Model file for the job. Use its own axes, mm. Give positions to 0.01 mm unless a question says otherwise; leave off trailing zeros. Order: outer loops, then holes, each group sorted by start corner. A loop starts at its lowest first (then second) coordinate and runs counter-clockwise, first axis right, second up. Notation, with made-up numbers: (8, 79.25) - (41, 79.25) arc R10 ccw to (41, 92.25) - close; hole circle Ø1 at (23, 16.25). An arc over 180 degrees is marked (long way). Use CSV: the item, a comma, the result in double quotes. Start each with the question number.
(1) Band-saw the part on B-B, the plane z = 0. Give the cut face in (x, y), then the cut area to 3 significant figures.
(2) Band-saw the part on A-A, the plane y = 20.25. Give the cut face in (x, z), then the cut area to 3 significant figures.
(3) Pull direction Z, two halves, no side cores. Call faces 1 (the flat face through (98.6, 22.181, -39.263)), 2 (the cylindrical face through (224.31, 22.27, -0.75)), 3 (the flat face through (89, 19.05, -1)): +Z half, -Z half, draft (parallel to the pull), parting line (faces both ways), or undercut.
(4) Probe L1, parallel to X at y = 20.5, z = 0; L2, parallel to Z at x = 200, y = 19.75; L3, parallel to Z at x = 121, y = 22.25. List the from-to ranges inside material, lowest first.
(5) Drop flat-ended pins along their axis: pin 1 Ø3 at (x, z) = (-47.57, 0) entering from -Y; pin 2 Ø1.5 at (y, z) = (21, 28) entering from -X; pin 3 Ø3 at (x, y) = (95.5, 24.5) entering from -Z; pin 4 Ø3 at (x, y) = (-7.5, 23.5) entering from -Z. Give the stop position or say it passes through.
(6) Band-saw the part on D-D, the plane z = 34. Give the cut face in (x, y), then the cut area to 3 significant figures.
(7) Band-saw the part on C-C, the plane x = 32. Give the cut face in (y, z), then the cut area to 3 significant figures.
from build123d import *

# Parameters (mm, degrees)
BOSS_EXTRUDE1_DEPTH = 25.4
SKETCH3_R           = 2.5
CUT_EXTRUDE2_DEPTH  = 25.4
CUT_EXTRUDE3_DEPTH  = 19.05
SKETCH4_R           = 4.5
CUT_EXTRUDE4_DEPTH  = 19.05


with BuildPart() as part:
    # Sketch1 → Boss-Extrude1 (new body)
    with BuildSketch(Plane(origin=(0, 0, 0), x_dir=(1, 0, 0), z_dir=(0, 1, 0))):
        with BuildLine():
            Line((0, 50.892363224), (200.000108, 27.30276997))
            ThreePointArc((200.000108, 27.30276997), (225.337078532, 1.965799438), (200.000108, -23.371171094))
            Line((200.000108, -23.371171094), (0, -50.892363224))
            ThreePointArc((0, -50.892363224), (-50.892363224, 0), (0, 50.892363224))
        make_face()
    extrude(amount=BOSS_EXTRUDE1_DEPTH)

    # Sketch3 → Cut-Extrude2 (cut)
    with BuildSketch(Plane(origin=(0, 25.4, 0), x_dir=(1, 0, 0), z_dir=(0, 1, 0))):
        with Locations((-47.56908022, 0)):
            Circle(SKETCH3_R)
        with Locations((221.926143204, 0)):
            Circle(SKETCH3_R)
    extrude(amount=-CUT_EXTRUDE2_DEPTH, mode=Mode.SUBTRACT)

    # Sketch1<3> → Cut-Extrude3 (cut)
    with BuildSketch(Plane(origin=(0, 0, 0), x_dir=(1, 0, 0), z_dir=(0, 1, 0))):
        with BuildLine():
            Line((0, 50.892363224), (200.000108, 27.30276997))
            ThreePointArc((200.000108, 27.30276997), (225.337078532, 1.965799438), (200.000108, -23.371171094))
            Line((200.000108, -23.371171094), (0, -50.892363224))
            ThreePointArc((0, -50.892363224), (-50.892363224, 0), (0, 50.892363224))
        make_face()
    extrude(amount=CUT_EXTRUDE3_DEPTH, mode=Mode.SUBTRACT)

    # Sketch4 → Cut-Extrude4 (cut)
    with BuildSketch(Plane(origin=(0, 25.4, 0), x_dir=(1, 0, 0), z_dir=(0, 1, 0))):
        Circle(SKETCH4_R)
        with Locations((200.000108, 0)):
            Circle(SKETCH4_R)
    extrude(amount=-CUT_EXTRUDE4_DEPTH, mode=Mode.SUBTRACT)


solid = part.part
Answer block:
1,outline,"(-50.89, 19.05) - (-50.07, 19.05) - (-50.07, 25.4) - (-50.89, 25.4) - close; (-45.07, 19.05) - (-4.5, 19.05) - (-4.5, 25.4) - (-45.07, 25.4) - close; (4.5, 19.05) - (195.5, 19.05) - (195.5, 25.4) - (4.5, 25.4) - close; (204.5, 19.05) - (219.43, 19.05) - (219.43, 25.4) - (204.5, 25.4) - close; (224.43, 19.05) - (225.26, 19.05) - (225.26, 25.4) - (224.43, 25.4) - close"
1,area,"1,580 mm2"
2,outline,"(0, -50.89) - (200, -27.3) arc R25.34 ccw to (200, 23.37) - (0, 50.89) arc R50.89 ccw to start; hole circle Ø5 at (-47.57, 0); hole circle Ø9 at (0, 0); hole circle Ø9 at (200, 0); hole circle Ø5 at (221.93, 0)"
2,area,"20,200 mm2"
3,face 1,"-Z half"
3,face 2,"undercut"
3,face 3,"draft"
4,L1,"x = -50.89 to -50.07, -45.07 to -4.5, 4.5 to 195.5, 204.5 to 219.43, 224.43 to 225.26"
4,L2,"z = -27.3 to -4.5, 4.5 to 23.37"
4,L3,"z = -36.62 to 34.24"
5,pin 1,"passes through"
5,pin 2,"stops at x = -42.98"
5,pin 3,"stops at z = -39.81"
5,pin 4,"stops at z = -50.54"
6,outline,"(-37.87, 19.05) - (122.76, 19.05) - (122.76, 25.4) - (-37.87, 25.4) - close"
6,area,"1,020 mm2"
7,outline,"(19.05, -47.12) - (25.4, -47.12) - (25.4, 46.49) - (19.05, 46.49) - close"
7,area,"594 mm2"
